from build123d import *

# Parameters (mm, degrees)
IZIM1_R                     = 22.5
Y_KSEKLIK_EKSTR_ZYON1_DEPTH = 60
IZIM2_R                     = 40
IZIM2_R_2                   = 22.5
Y_KSEKLIK_EKSTR_ZYON2_DEPTH = 5
IZIM3_W                     = 50
IZIM3_H                     = 50
Y_KSEKLIK_EKSTR_ZYON3_DEPTH = 50
IZIM4_R                     = 25
Y_KSEKLIK_EKSTR_ZYON4_DEPTH = 27.5
IZIM5_R                     = 8
KES_EKSTR_ZYON1_DEPTH       = 68.5


with BuildPart() as part:
    # Çizim1 → Yükseklik-Ekstrüzyon1 (new body)
    with BuildSketch(Plane(origin=(0, 0, 0), x_dir=(1, 0, 0), z_dir=(0, 1, 0))):
        Circle(IZIM1_R)
    extrude(amount=Y_KSEKLIK_EKSTR_ZYON1_DEPTH)

    # Çizim2 → Yükseklik-Ekstrüzyon2 (add)
    with BuildSketch(Plane(origin=(0, 60, 0), x_dir=(1, 0, 0), z_dir=(0, 1, 0))):
        Circle(IZIM2_R)
        Circle(IZIM2_R_2, mode=Mode.SUBTRACT)
    extrude(amount=-Y_KSEKLIK_EKSTR_ZYON2_DEPTH)

    # Çizim3 → Yükseklik-Ekstrüzyon3 (add)
    with BuildSketch(Plane(origin=(0, 60, 0), x_dir=(1, 0, 0), z_dir=(0, 1, 0))):
        Rectangle(IZIM3_W, IZIM3_H)
    extrude(amount=Y_KSEKLIK_EKSTR_ZYON3_DEPTH)

    # Çizim4 → Yükseklik-Ekstrüzyon4 (add, symmetric)
    with BuildSketch(Plane.XY):
        with Locations((0, 110)):
            Circle(IZIM4_R)
    extrude(amount=Y_KSEKLIK_EKSTR_ZYON4_DEPTH, both=True)

    # Çizim5 → Kes-Ekstrüzyon1 (cut, through all)
    with BuildSketch(Plane.XY.offset(27.5)):
        with Locations((0, 110)):
            Circle(IZIM5_R)
    extrude(amount=-KES_EKSTR_ZYON1_DEPTH, mode=Mode.SUBTRACT)


solid = part.part
Input: part model. Units: mm. Frame: model coordinates. A direction names the side the tool comes from. Coordinates: 2 decimals unless noted, no trailing zeros. Write each loop counter-clockwise with the first axis right and the second up, starting at its lowest first coordinate (ties: lowest second). Pieces come first, ordered by that corner, then holes. Notation, with made-up numbers: M 73.5,38 L 102.5,38 A11 ccw 102.5,42 Z; hole C 2,54 d11. An arc over 180 degrees is marked long. Answer as a JSON object with one key per item and string values. Group by question number.
(1) Contact query for flat-ended pins moving along their axis: P1, Ø2, axis at x = 15, z = 11, coming from the +Y side; P2, Ø25, axis at x = 5, y = 88.5, coming from the -Z side; P3, Ø15, axis at y = 89, z = -10.5, coming from the +X side; P4, Ø4, axis at y = 111, z = 31, coming from the -X side (1 decimal). Output: stop coordinate, or through.
(2) Mould query, pull axis Y, two halves, no side actions, for faces 4 (the face through (0, 74, 25)), 5 (the face through (-6, 116, 27.5)), 6 (the face through (17, 55, 17)). Classes: pulls with the +Y half, pulls with the -Y half, needs draft (parallel to the pull), parting line crosses it, or undercut.
(3) Set-up query: faces 1 (the face through (25, 85, 0)), 2 (the face through (-6, 116, -27.5)), 3 (the face through (26, 60, -1)). Return all of +Z, -Z, +X, -X, +Y, -Y with unobstructed straight access to the full face (end or side cutting, diameter ignored); none if empty.
(4) Ray query, line 1 along Y through (x, z) = (0, 10); line 2 along X through (y, z) = (105.5, -26); line 3 along X through (y, z) = (87.5, -3.5). Return the intervals inside material, ascending. Write a range as [from, to].
(5) Section C-C on y = 115. Output: boundary loops of the cut face in (x, z) (3 decimals), plus the area to 3 significant figures.
(6) Section A-A on x = 0. Output: boundary loops of the cut face in (y, z).
(7) Section B-B on z = 0. Output: boundary loops of the cut face in (x, y).
(8) Section D-D on x = 20. Output: boundary loops of the cut face in (y, z).
Result set:
{
 "1": {"P1": "stops at y = 130.71", "P2": "stops at z = -27.5", "P3": "stops at x = 25", "P4": "passes through"},
 "2": {"face 4": "undercut", "face 5": "needs draft", "face 6": "pulls with the -Y half"},
 "3": {"face 1": "+Z, -Z, +X, +Y", "face 2": "-Z, +X, -X, +Y", "face 3": "none"},
 "4": {"line 1": "y = [0, 102], [118, 135]", "line 2": "x = [-24.59, -6.61], [6.61, 24.59]", "line 3": "x = [-25, 25]"},
 "5": {"outline": "M -24.495,-27.5 L -6.245,-27.5 L -6.245,27.5 L -24.495,27.5 Z; M 6.245,-27.5 L 24.495,-27.5 L 24.495,27.5 L 6.245,27.5 Z", "area": "2,010 mm2"},
 "6": {"outline": "M 0,-22.5 L 55,-22.5 L 55,-40 L 60,-40 L 60,-25 L 85,-25 L 85,-27.5 L 102,-27.5 L 102,27.5 L 85,27.5 L 85,25 L 60,25 L 60,40 L 55,40 L 55,22.5 L 0,22.5 Z; M 118,-27.5 L 135,-27.5 L 135,27.5 L 118,27.5 Z"},
 "7": {"outline": "M -40,55 L -22.5,55 L -22.5,0 L 22.5,0 L 22.5,55 L 40,55 L 40,60 L 25,60 L 25,110 A25 ccw -25,110 L -25,60 L -40,60 Z; hole C 0,110 d16"},
 "8": {"outline": "M 0,-10.31 L 55,-10.31 L 55,-34.64 L 60,-34.64 L 60,-25 L 95,-25 L 95,-27.5 L 125,-27.5 L 125,27.5 L 95,27.5 L 95,25 L 60,25 L 60,34.64 L 55,34.64 L 55,10.31 L 0,10.31 Z"}
}
